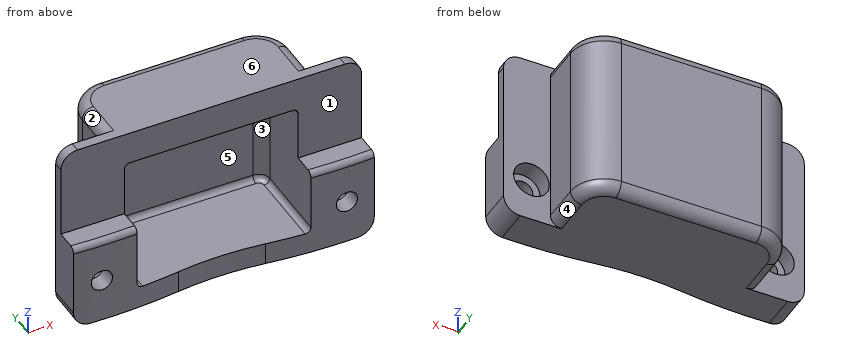
from build123d import *

# Parameters (mm, degrees)
EXTRUDE_1_DEPTH     = 4
CUT_EXTRUDE_1_REACH = 19.27
SKETCH_2_R          = 0.95
SKETCH_5_W          = 15.6
SKETCH_5_H          = 6
CUT_EXTRUDE_2_DEPTH = 8.5
CUT_EXTRUDE_4_DEPTH = 19.607794066
EXTRUDE_2_DEPTH     = 8
SKETCH_12_W         = 15.6
SKETCH_12_H         = 3
EXTRUDE_3_DEPTH     = 5.9
SKETCH_13_R         = 1.6
CUT_EXTRUDE_5_DEPTH = 1.6
FILLET_1_R          = 3
FILLET_2_R          = 1
FILLET_3_R          = 1.5
FILLET_4_R          = 1
FILLET_5_R          = 0.5
FILLET_6_R          = 0.5


with BuildPart() as part:
    # 草图1 → 凸台-拉伸1 (new, symmetric)
    with BuildSketch(Plane.XY):
        Polygon((-13.5, 0), (-13.5, 3.5), (-9.3, 3.5), (-9.3, 10), (9.3, 10), (9.3, 3.5), (13.5, 3.5), (13.5, 0), align=None)
    extrude(amount=EXTRUDE_1_DEPTH, both=True)

    # 草图2 → 切除-拉伸1 (cut, up to next)
    with BuildSketch(Plane.XZ, mode=Mode.PRIVATE) as cut_extrude_1_sk1:
        with Locations((-11, 0)):
            Circle(SKETCH_2_R)
    cut_extrude_1_tool1 = extrude(cut_extrude_1_sk1.sketch, amount=-CUT_EXTRUDE_1_REACH, mode=Mode.PRIVATE) & part.part
    # 草图2 → 切除-拉伸1 (cut, up to next)
    with BuildSketch(Plane.XZ, mode=Mode.PRIVATE) as cut_extrude_1_sk2:
        with Locations((11, 0)):
            Circle(SKETCH_2_R)
    cut_extrude_1_tool2 = extrude(cut_extrude_1_sk2.sketch, amount=-CUT_EXTRUDE_1_REACH, mode=Mode.PRIVATE) & part.part
    add(cut_extrude_1_tool1.solids().sort_by_distance((-11, 0, 0))[0], mode=Mode.SUBTRACT)
    add(cut_extrude_1_tool2.solids().sort_by_distance((11, 0, 0))[0], mode=Mode.SUBTRACT)

    # 草图5 → 切除-拉伸2 (cut)
    with BuildSketch(Plane(origin=(0, 0, 0), x_dir=(-1, 0, 0), z_dir=(0, -1, 0))):
        with Locations((0, -1)):
            Rectangle(SKETCH_5_W, SKETCH_5_H)
    extrude(amount=-CUT_EXTRUDE_2_DEPTH, mode=Mode.SUBTRACT)

    # 草图8 → 切除-拉伸4 (cut, through all)
    with BuildSketch(Plane(origin=(0, 0, -4), x_dir=(-1, 0, 0), z_dir=(0, 0, -1))):
        with BuildLine():
            Line((-18.493720414, 0.960055854), (-18.493720414, -4.039944146))
            Line((-18.493720414, -4.039944146), (18.493720414, -4.039944146))
            Line((18.493720414, -4.039944146), (18.493720414, 0.960055854))
            ThreePointArc((18.493720414, 0.960055854), (11.217877694, 0.317576425), (3.926064508, 0.741990812))
            ThreePointArc((3.926064508, 0.741990812), (0, 1), (-3.926064508, 0.741990812))
            ThreePointArc((-3.926064508, 0.741990812), (-11.217877694, 0.317576425), (-18.493720414, 0.960055854))
        make_face()
    extrude(amount=-CUT_EXTRUDE_4_DEPTH, mode=Mode.SUBTRACT)

    # 草图11 → 凸台-拉伸2 (add)
    with BuildSketch(Plane.XY.offset(4)):
        Polygon((13.5, 2.6), (7.8, 2.6), (7.8, 8.5), (-7.8, 8.5), (-7.8, 2.6), (-13.5, 2.6), (-13.5, 3.5), (-9.3, 3.5), (-9.3, 10), (9.3, 10), (9.3, 3.5), (13.5, 3.5), align=None)
    extrude(amount=EXTRUDE_2_DEPTH)

    # 草图12 → 凸台-拉伸3 (add)
    with BuildSketch(Plane.XZ.offset(-8.5)):
        with Locations((0, 10.5)):
            Rectangle(SKETCH_12_W, SKETCH_12_H)
    extrude(amount=EXTRUDE_3_DEPTH)

    # 草图13 → 切除-拉伸5 (cut)
    with BuildSketch(Plane(origin=(0, 3.5, 0), x_dir=(1, 0, 0), z_dir=(0, 1, 0))):
        with Locations(Location((-11, 0, 0), (0, 0, 270))):
            Circle(SKETCH_13_R)
        with Locations(Location((11, 0, 0), (0, 0, 270))):
            Circle(SKETCH_13_R)
    extrude(amount=-CUT_EXTRUDE_5_DEPTH, mode=Mode.SUBTRACT)

    # 圆角1
    fillet_1_edges = [part.edges().sort_by_distance(p)[0] for p in [
        (-9.3, 10, 4),
        (9.3, 10, 4),
    ]]
    fillet(fillet_1_edges, radius=FILLET_1_R)

    # 圆角2
    fillet_2_edges = [part.edges().sort_by_distance(p)[0] for p in [
        (7.8, 8.5, 3.5),
        (-7.8, 8.5, 3.5),
    ]]
    fillet(fillet_2_edges, radius=FILLET_2_R)

    # 圆角3
    fillet_3_edges = [part.edges().sort_by_distance(p)[0] for p in [
        (13.5, 3.05, 12),
        (-13.5, 3.05, 12),
        (13.5, 1.951949488, -4),
        (-13.5, 1.951949488, -4),
    ]]
    fillet(fillet_3_edges, radius=FILLET_3_R)

    # 圆角4
    fillet_4_edges = [part.edges().sort_by_distance(p)[0] for p in [
        (9.3, 5.25, -4),
        (9.3, 5.25, 12),
        (0, 10, -4),
        (0, 10, 12),
        (-9.3, 5.25, -4),
        (-8.421320344, 9.121320344, -4),
        (8.421320344, 9.121320344, -4),
        (-9.3, 5.25, 12),
        (-8.421320344, 9.121320344, 12),
        (8.421320344, 9.121320344, 12),
    ]]
    fillet(fillet_4_edges, radius=FILLET_4_R)

    # 圆角5
    fillet_5_edges = [part.edges().sort_by_distance(p)[0] for p in [
        (10.650293934, 0.312302345, 4),
        (-10.650293934, 0.312302345, 4),
    ]]
    fillet(fillet_5_edges, radius=FILLET_5_R)

    # 圆角6
    fillet_6_edges = [part.edges().sort_by_distance(p)[0] for p in [
        (7.8, 5.05, 9),
        (-7.8, 5.05, 9),
        (-7.8, 3.941644472, -2),
        (0, 8.5, 9),
        (7.507106781, 8.207106781, 9),
        (-7.507106781, 8.207106781, 9),
        (0, 8.5, -2),
        (7.8, 3.941644472, -2),
        (7.507106781, 8.207106781, -2),
        (-7.507106781, 8.207106781, -2),
    ]]
    fillet(fillet_6_edges, radius=FILLET_6_R)


solid = part.part
Build history of the part. All positions in model axes, mm. Face numbers are marked on the shaded views. A direction names the side the tool comes from. Round coordinates to 2 decimals unless told otherwise and drop trailing zeros. Loops run counter-clockwise (first coordinate to the right, second up) from the corner with the lowest first, then second, coordinate; pieces in that order, holes last. Notation, with made-up numbers: (29, 36) -> (79, 36) arc R33 ccw to (79, 70) -> close; hole circle Ø10 at (22, 47). An arc over 180 degrees is marked (long way). One line per item, written item: value. Start each with the question number.
Q1. Drop flat-ended pins along their axis: pin 1 Ø5.5 at (x, z) = (-10.5, 7.5) entering from +Y; pin 2 Ø1.6 at (x, z) = (11, 0.5) entering from +Y; pin 3 Ø2 at (y, z) = (5.5, 5) entering from -X. Give the stop position or say it passes through.
Q2. Cut at B-B on z = 0.5. Count the separate pieces of the cut face and the enclosed holes in it, plus the area to 3 significant figures.
Q3. Cut at D-D on z = 4.75. List the corners of the cut face in (x, y), plus the area to 3 significant figures.
Q4. Two-plate mould, pull along X, no slides. Class the marked faces 4, 5 and 6: released by +X, released by -X, zero draft, split by the parting line, or undercut.
Q5. Probe line 1 along X through (y, z) = (2.25, 0); line 2 along Z through (x, y) = (-11, 1.25); line 3 along X through (y, z) = (6, 5). List the from-to ranges inside material, lowest first.
Q6. Cut at A-A on y = 1.5. List the corners of the cut face in (x, z).
Q7. Cut at C-C on y = 3. List the corners of the cut face in (x, z).
Q8. 3-axis set-ups, long thin cutter, end or side, ignore diameter. For the marked faces 1, 2 and 3: which of +Z, -Z, +X, -X, +Y, -Y reach the whole face in a straight line?
Computed:
1. pin 1: y = 9.63
1. pin 2: y = 1.9
1. pin 3: x = -9.3
2. separate pieces: 3
2. enclosed holes: 0
2. area: 60.7 mm²
3. outline: (-13.5, 2.6) -> (-7.8, 2.6) -> (-7.8, 7.5) arc R1 cw to (-6.8, 8.5) -> (6.8, 8.5) arc R1 cw to (7.8, 7.5) -> (7.8, 2.6) -> (13.5, 2.6) -> (13.5, 3.5) -> (9.3, 3.5) -> (9.3, 7) arc R3 ccw to (6.3, 10) -> (-6.3, 10) arc R3 ccw to (-9.3, 7) -> (-9.3, 3.5) -> (-13.5, 3.5) -> close
3. area: 49.7 mm²
4. face 4: released by +X
4. face 5: undercut
4. face 6: zero draft
5. line 1: -13.5 to -12.6, -9.4 to -7.8, 7.8 to 9.4, 12.6 to 13.5
5. line 2: -4 to -0.95, 0.95 to 4
5. line 3: -9.3 to -7.8, 7.8 to 9.3
6. outline: (-13.5, -2.5) arc R1.5 ccw to (-12, -4) -> (12, -4) arc R1.5 ccw to (13.5, -2.5) -> (13.5, 4) -> (7.8, 4) -> (7.8, -1.5) arc R0.5 cw to (7.3, -2) -> (-7.3, -2) arc R0.5 cw to (-7.8, -1.5) -> (-7.8, 4) -> (-13.5, 4) -> close; hole circle Ø1.9 at (-11, 0); hole circle Ø1.9 at (11, 0)
7. outline: (-13.5, -2.5) arc R1.5 ccw to (-12, -4) -> (12, -4) arc R1.5 ccw to (13.5, -2.5) -> (13.5, 10.5) arc R1.5 ccw to (12, 12) -> (-12, 12) arc R1.5 ccw to (-13.5, 10.5) -> close; hole circle Ø3.2 at (-11, 0); hole (-7.8, -1.5) arc R0.5 ccw to (-7.3, -2) -> (7.3, -2) arc R0.5 ccw to (7.8, -1.5) -> (7.8, 8.5) arc R0.5 ccw to (7.3, 9) -> (-7.3, 9) arc R0.5 ccw to (-7.8, 8.5) -> close; hole circle Ø3.2 at (11, 0)
8. face 1: +Z, +X, -X, -Y
8. face 2: +Z, -X, +Y
8. face 3: -Y
